The listing builds one solid part. Answer for the finished solid, in the listing's coordinates (mm). A direction names the side the tool comes from. Give positions to 0.01 mm unless a question says otherwise; leave off trailing zeros. Write each loop counter-clockwise with the first axis right and the second up, starting at its lowest first coordinate (ties: lowest second). Pieces come first, ordered by that corner, then holes. Notation, with made-up numbers: M -0.75,78.25 L 41.25,78.25 A28 cw 41.25,112.25 Z; hole C 31,64.5 d4. An arc over 180 degrees is marked long. Return JSON: item names as keys, results as strings.
from build123d import *

# Parameters (mm, degrees)
SKETCH1_W           = 76.2
SKETCH1_H           = 114.3
BOSS_EXTRUDE1_DEPTH = 25.4


with BuildPart() as part:
    # Sketch1 → Boss-Extrude1 (new body)
    with BuildSketch(Plane(origin=(0, 0, 0), x_dir=(1, 0, 0), z_dir=(0, 1, 0))):
        Polygon((-76.2, 57.15), (76.2, 57.15), (0, 156.455773411), align=None)
        Rectangle(SKETCH1_W, SKETCH1_H)
        with BuildLine():
            ThreePointArc((25.4, 156.455773411), (-11.234132732, 179.236341045), (-15.462540297, 136.304598567))
            Line((-15.462540297, 136.304598567), (0, 156.455773411))
            Line((0, 156.455773411), (15.462540297, 136.304598567))
            ThreePointArc((15.462540297, 136.304598567), (22.780567635, 145.221640679), (25.4, 156.455773411))
        make_face()
        with BuildLine():
            Line((0, 156.455773411), (-15.462540297, 136.304598567))
            ThreePointArc((-15.462540297, 136.304598567), (0, 131.055773411), (15.462540297, 136.304598567))
            Line((15.462540297, 136.304598567), (0, 156.455773411))
        make_face()
    extrude(amount=BOSS_EXTRUDE1_DEPTH)


solid = part.part
Item 1: Given pin 1 Ø2 at (y, z) = (5.5, -38) entering from -X; pin 2 Ø7.5 at (x, y) = (66, 17) entering from +Z; pin 3 Ø4 at (x, y) = (-7.5, 12.5) entering from -Z, each flat-ended and moving along its own axis, determine where each tip first touches the part or whether it passes through.
Geometry results:
{"pin 1": "stops at x = -38.1", "pin 2": "stops at z = -57.15", "pin 3": "stops at z = -181.25"}
Item 2: Find the intervals of material crossed by line 1 (X direction, y = 13.75, z = -10); line 2 (X direction, y = 20, z = -115); line 3 (Z direction, x = -22, y = 14.5), in increasing order.
Geometry results:
{"line 1": "x = -38.1 to 38.1", "line 2": "x = -31.81 to 31.81", "line 3": "z = -169.15 to -143.76, -127.78 to 57.15"}
Item 3: A cutting plane is placed at D-D, the plane z = -159. Write down the section's boundary in (x, y), plus the area to 3 significant figures.
Geometry results:
{"outline": "M -25.27,0 L 25.27,0 L 25.27,25.4 L -25.27,25.4 Z", "area": "1,280 mm2"}
Item 4: Which of the six approach directions +Z, -Z, +X, -X, +Y, -Y give full straight-line access (tool end or side, diameter ignored) to faces 1 (the flat face through (-45.406, 12.522, -97.281)), 2 (the flat face through (38.1, 13, 1)), 3 (the flat face through (-1, 25.4, -64)), 4 (the flat face through (-57, 13, -57.15))?
Geometry results:
{"face 1": "-X, +Y, -Y", "face 2": "+Z, +X, +Y, -Y", "face 3": "+Z, -Z, +X, -X, +Y", "face 4": "+Z, -X, +Y, -Y"}
Item 5: A cutting plane is placed at B-B, the plane y = 5. Write down the section's boundary in (x, z), plus the area to 3 significant figures.
Geometry results:
{"outline": "M -76.2,-57.15 L -15.46,-136.3 A25.4 ccw long 15.46,-136.3 L 76.2,-57.15 L 38.1,-57.15 L 38.1,57.15 L -38.1,57.15 L -38.1,-57.15 Z", "area": "17,900 mm2"}
Item 6: A cutting plane is placed at C-C, the plane z = -40.5. Write down the section's boundary in (x, y).
Geometry results:
{"outline": "M -38.1,0 L 38.1,0 L 38.1,25.4 L -38.1,25.4 Z"}
Item 7: A cutting plane is placed at A-A, the plane x = -21.5. Write down the section's boundary in (y, z).
Geometry results:
{"outline": "M 0,-169.98 L 25.4,-169.98 L 25.4,-142.93 L 0,-142.93 Z; M 0,-128.44 L 25.4,-128.44 L 25.4,57.15 L 0,57.15 Z"}
